from build123d import *

# Parameters (mm, degrees)
F1_START = 3
F0_R     = 1.75
F1_DEPTH = 1.5
F2_START = 14.5
F2_DEPTH = 1.5
F3_R     = 1.25
F4_DEPTH = 3
F5_START = 4.5
F5_DEPTH = 10
F6_START = 16
F6_DEPTH = 3


with BuildPart() as f1:
    # F0 (on Top) → F1 (new body)
    with BuildSketch(Plane.XY.offset(F1_START)):
        with BuildLine():
            Line((15.25, 18), (-15.25, 18))
            ThreePointArc((-15.25, 18), (-17.1945436483, 17.1945436483), (-18, 15.25))
            Line((-18, 15.25), (-18, -15.25))
            ThreePointArc((-18, -15.25), (-17.1945436483, -17.1945436483), (-15.25, -18))
            Line((-15.25, -18), (15.25, -18))
            ThreePointArc((15.25, -18), (17.1945436483, -17.1945436483), (18, -15.25))
            Line((18, -15.25), (18, 15.25))
            ThreePointArc((18, 15.25), (17.1945436483, 17.1945436483), (15.25, 18))
        make_face()
        with Locations((-15.25, -15.25)):
            Circle(F0_R, mode=Mode.SUBTRACT)
        with Locations((15.25, -15.25)):
            Circle(F0_R, mode=Mode.SUBTRACT)
        with Locations((-15.25, 15.25)):
            Circle(F0_R, mode=Mode.SUBTRACT)
        with Locations((15.25, 15.25)):
            Circle(F0_R, mode=Mode.SUBTRACT)
    extrude(amount=F1_DEPTH)

    # F3 (on Top) → F4 (join)
    with BuildSketch(Plane.XY):
        Polygon((-13.5179491924, -18.25), (-11.7858983849, -15.25), (-13.5179491924, -12.25), (-16.9820508076, -12.25), (-18.7141016151, -15.25), (-16.9820508076, -18.25), align=None)
        with Locations((-15.25, -15.25)):
            Circle(F3_R, mode=Mode.SUBTRACT)
        Polygon((18.7141016151, -15.25), (16.9820508076, -12.25), (13.5179491924, -12.25), (11.7858983849, -15.25), (13.5179491924, -18.25), (16.9820508076, -18.25), align=None)
        with Locations((15.25, -15.25)):
            Circle(F3_R, mode=Mode.SUBTRACT)
        Polygon((13.5179491924, 18.25), (11.7858983849, 15.25), (13.5179491924, 12.25), (16.9820508076, 12.25), (18.7141016151, 15.25), (16.9820508076, 18.25), align=None)
        with Locations((15.25, 15.25)):
            Circle(F3_R, mode=Mode.SUBTRACT)
        Polygon((-13.5179491924, 12.25), (-11.7858983849, 15.25), (-13.5179491924, 18.25), (-16.9820508076, 18.25), (-18.7141016151, 15.25), (-16.9820508076, 12.25), align=None)
        with Locations((-15.25, 15.25)):
            Circle(F3_R, mode=Mode.SUBTRACT)
    extrude(amount=F4_DEPTH)



with BuildPart() as f2:
    # F0 (on Top) → F2 (new body)
    with BuildSketch(Plane.XY.offset(F2_START)):
        with BuildLine():
            Line((15.25, 18), (-15.25, 18))
            ThreePointArc((-15.25, 18), (-17.1945436483, 17.1945436483), (-18, 15.25))
            Line((-18, 15.25), (-18, -15.25))
            ThreePointArc((-18, -15.25), (-17.1945436483, -17.1945436483), (-15.25, -18))
            Line((-15.25, -18), (15.25, -18))
            ThreePointArc((15.25, -18), (17.1945436483, -17.1945436483), (18, -15.25))
            Line((18, -15.25), (18, 15.25))
            ThreePointArc((18, 15.25), (17.1945436483, 17.1945436483), (15.25, 18))
        make_face()
        with Locations((-15.25, -15.25)):
            Circle(F0_R, mode=Mode.SUBTRACT)
        with Locations((15.25, -15.25)):
            Circle(F0_R, mode=Mode.SUBTRACT)
        with Locations((-15.25, 15.25)):
            Circle(F0_R, mode=Mode.SUBTRACT)
        with Locations((15.25, 15.25)):
            Circle(F0_R, mode=Mode.SUBTRACT)
    extrude(amount=F2_DEPTH)


with BuildPart() as f1_1:
    add(f1.part)

    add(f2.part)  # F5 merges F2
    # F3 (on Top) → F5 (join)
    with BuildSketch(Plane.XY.offset(F5_START)):
        Polygon((-13.5179491924, -18.25), (-11.7858983849, -15.25), (-13.5179491924, -12.25), (-16.9820508076, -12.25), (-18.7141016151, -15.25), (-16.9820508076, -18.25), align=None)
        with Locations((-15.25, -15.25)):
            Circle(F3_R, mode=Mode.SUBTRACT)
        Polygon((18.7141016151, -15.25), (16.9820508076, -12.25), (13.5179491924, -12.25), (11.7858983849, -15.25), (13.5179491924, -18.25), (16.9820508076, -18.25), align=None)
        with Locations((15.25, -15.25)):
            Circle(F3_R, mode=Mode.SUBTRACT)
        Polygon((13.5179491924, 18.25), (11.7858983849, 15.25), (13.5179491924, 12.25), (16.9820508076, 12.25), (18.7141016151, 15.25), (16.9820508076, 18.25), align=None)
        with Locations((15.25, 15.25)):
            Circle(F3_R, mode=Mode.SUBTRACT)
        Polygon((-13.5179491924, 12.25), (-11.7858983849, 15.25), (-13.5179491924, 18.25), (-16.9820508076, 18.25), (-18.7141016151, 15.25), (-16.9820508076, 12.25), align=None)
        with Locations((-15.25, 15.25)):
            Circle(F3_R, mode=Mode.SUBTRACT)
    extrude(amount=F5_DEPTH)

    # F3 (on Top) → F6 (join)
    with BuildSketch(Plane.XY.offset(F6_START)):
        Polygon((-13.5179491924, -18.25), (-11.7858983849, -15.25), (-13.5179491924, -12.25), (-16.9820508076, -12.25), (-18.7141016151, -15.25), (-16.9820508076, -18.25), align=None)
        with Locations((-15.25, -15.25)):
            Circle(F3_R, mode=Mode.SUBTRACT)
        Polygon((18.7141016151, -15.25), (16.9820508076, -12.25), (13.5179491924, -12.25), (11.7858983849, -15.25), (13.5179491924, -18.25), (16.9820508076, -18.25), align=None)
        with Locations((15.25, -15.25)):
            Circle(F3_R, mode=Mode.SUBTRACT)
        Polygon((13.5179491924, 18.25), (11.7858983849, 15.25), (13.5179491924, 12.25), (16.9820508076, 12.25), (18.7141016151, 15.25), (16.9820508076, 18.25), align=None)
        with Locations((15.25, 15.25)):
            Circle(F3_R, mode=Mode.SUBTRACT)
        Polygon((-13.5179491924, 12.25), (-11.7858983849, 15.25), (-13.5179491924, 18.25), (-16.9820508076, 18.25), (-18.7141016151, 15.25), (-16.9820508076, 12.25), align=None)
        with Locations((-15.25, 15.25)):
            Circle(F3_R, mode=Mode.SUBTRACT)
    extrude(amount=F6_DEPTH)


solid = f1_1.part
Geometry: final body of the model. Coordinates: model frame, mm. A direction names the side the tool comes from. Round coordinates to 2 decimals unless told otherwise and drop trailing zeros. Loops run counter-clockwise (first coordinate to the right, second up) from the corner with the lowest first, then second, coordinate; pieces in that order, holes last.
Q1. Material intervals for L1, parallel to Y at x = 15.25, z = 3.6; L2, parallel to Y at x = 15.25, z = 10; L3, parallel to Z at x = 3, y = 6.5, sorted ascending.
Q2. Section A-A on z = 17. Return loops of the section in (x, y), plus the area to 3 significant figures.
Q3. Pin query (flat end, axial travel): P1, Ø2, axis at x = 10, y = 9, coming from the +Z side; P2, Ø3, axis at x = 9, y = -9.5, coming from the -Z side; P3, Ø3, axis at x = -16, y = 16, coming from the +Z side; P4, Ø8, axis at y = -13.5, z = 10, coming from the +X side. Return the tip coordinate at first contact, or that it passes through.
Q4. Pull-direction query (Z, two-part tool) for faces 1 (the flat face through (-13.8, 15.3, 19)), 2 (the flat face through (-12.64, -13.77, 9.43)), 3 (the cylindrical face through (15.09, -14.01, 9.43)); classes: released by +Z, released by -Z, zero draft, split by the parting line, or undercut.
Q5. Section B-B on x = 0. Return loops of the section in (y, z), plus the area to 3 significant figures.
Q6. Access query for faces 4 (the flat face through (-15, 12.25, 17)), 5 (the flat face through (14, 16, 4.5)), 6 (the flat face through (-17.2, -17.4, 16)), 7 (the flat face through (-17.2, 17.4, 3)). Directions: +Z, -Z, +X, -X, +Y, -Y. A direction counts if a zero-diameter tool reaches every point of the face in a straight line with its end or side. Return the directions, or none.
Evaluation:
1. L1: y = -18 to -17, -13.5 to 13.5, 17 to 18
1. L2: y = -18.25 to -16.5, -14 to -12.25, 12.25 to 14, 16.5 to 18.25
1. L3: z = 3 to 4.5, 14.5 to 16
2. outline: (-18.71, -15.25) - (-16.98, -18.25) - (-13.52, -18.25) - (-11.79, -15.25) - (-13.52, -12.25) - (-16.98, -12.25) - close; (-18.71, 15.25) - (-16.98, 12.25) - (-13.52, 12.25) - (-11.79, 15.25) - (-13.52, 18.25) - (-16.98, 18.25) - close; (11.79, -15.25) - (13.52, -18.25) - (16.98, -18.25) - (18.71, -15.25) - (16.98, -12.25) - (13.52, -12.25) - close; (11.79, 15.25) - (13.52, 12.25) - (16.98, 12.25) - (18.71, 15.25) - (16.98, 18.25) - (13.52, 18.25) - close; hole circle Ø2.5 at (-15.25, -15.25); hole circle Ø2.5 at (-15.25, 15.25); hole circle Ø2.5 at (15.25, -15.25); hole circle Ø2.5 at (15.25, 15.25)
2. area: 105 mm2
3. P1: stops at z = 16
3. P2: stops at z = 3
3. P3: stops at z = 19
3. P4: stops at x = 18.71
4. face 1: released by +Z
4. face 2: undercut
4. face 3: zero draft
5. outline: (-18, 3) - (18, 3) - (18, 4.5) - (-18, 4.5) - close; (-18, 14.5) - (18, 14.5) - (18, 16) - (-18, 16) - close
5. area: 108 mm2
6. face 4: +Z, +X, -X
6. face 5: none
6. face 6: -X, -Y
6. face 7: -X, +Y
